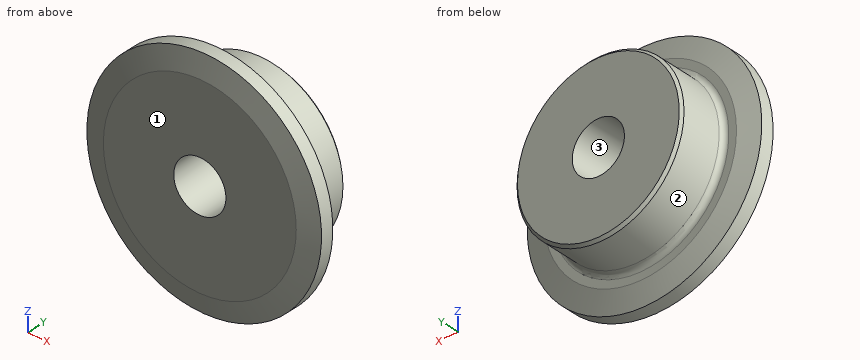
from build123d import *

# Parameters (mm, degrees)
F0_W     = 28.4
F0_H     = 40.5
F0_H_2   = 68.75
F0_W_2   = 59.1
F2_R     = 6.25
F3_SIZE  = 3.125
F4_SIZE2 = 25
F4_SIZE  = 6.2


with BuildPart() as f1:
    # F0 (on Right) → F1 (revolve)
    with BuildSketch(Plane.YZ):
        with Locations((14.2, 120.25)):
            Rectangle(F0_W, F0_H)
        with Locations((14.2, 65.625)):
            Rectangle(F0_W, F0_H_2)
        with Locations((57.95, 65.625)):
            Rectangle(F0_W_2, F0_H_2)
    revolve(axis=Axis((0, 43.75, 0), (0, 1, 0)))

    # F2
    f2_edges = [f1.edges().sort_by_distance(p)[0] for p in [
        (0, 28.4, -100),
    ]]
    fillet(f2_edges, radius=F2_R)

    # F3
    f3_edges = [f1.edges().sort_by_distance(p)[0] for p in [
        (0, 87.5, -100),
    ]]
    chamfer(f3_edges, length=F3_SIZE)

    # F4
    f4_edges = [f1.edges().sort_by_distance(p)[0] for p in [
        (0, 0, -140.5),
        (0, 28.4, -140.5),
    ]]
    f4_side = f1.faces().sort_by_distance((0, 14.2, -140.5))[0]
    chamfer(f4_edges, length=F4_SIZE, length2=F4_SIZE2, reference=f4_side)


solid = f1.part
Check sheet for the modelled part. Datum: model origin and axes. Units: mm. Face numbers are marked on the shaded views. Coordinates: 2 decimals unless noted, no trailing zeros. Write each loop counter-clockwise with the first axis right and the second up, starting at its lowest first coordinate (ties: lowest second). Pieces come first, ordered by that corner, then holes.
Item 1: Cross-section at B-B on z = 0. Record the boundary of the cut face in (x, y) (3 decimals), then the cut area to 3 significant figures.
Numbers:
outline: (-140.5, 6.2) - (-115.5, 0) - (-31.25, 0) - (-31.25, 87.5) - (-96.875, 87.5) - (-100, 84.375) - (-100, 34.65) arc R6.25 cw to (-106.25, 28.4) - (-115.5, 28.4) - (-140.5, 22.2) - close; (31.25, 0) - (115.5, 0) - (140.5, 6.2) - (140.5, 22.2) - (115.5, 28.4) - (106.25, 28.4) arc R6.25 cw to (100, 34.65) - (100, 84.375) - (96.875, 87.5) - (31.25, 87.5) - close
area: 14,000 mm2
Item 2: Mould release check, pull along X, two halves, no side actions. Record for the marked faces 1, 2 and 3: released by +X, released by -X, zero draft, split by the parting line, or undercut.
Numbers:
face 1: zero draft
face 2: split by the parting line
face 3: undercut
Item 3: Depth check by flat-ended pin: pin 1 Ø4 at (y, z) = (78, -92) entering from -X; pin 2 Ø12 at (x, y) = (-22.5, 70.5) entering from +Z; pin 3 Ø3 at (x, z) = (92.5, -83) entering from -Y. Enter the tip coordinate at first touch or a pass-through.
Numbers:
pin 1: stops at x = -43.59
pin 2: stops at z = 98.63
pin 3: stops at y = 1.81
Item 4: Cross-section at C-C on y = 39. Record the boundary of the cut face in (x, z).
Numbers:
outline: circle Ø200 at (0, 0); hole circle Ø62.5 at (0, 0)
Item 5: Scan lines: probe 1 along X at (y, z) = (69, 0); probe 2 along X at (y, z) = (16, 1.5); probe 3 along Y at (x, z) = (58, -121.5). Record each from-to range of solid material in increasing order.
Numbers:
probe 1: x = -100 to -31.25, 31.25 to 100
probe 2: x = -140.49 to -31.21, 31.21 to 140.49
probe 3: y = 4.75 to 23.65
Item 6: Cross-section at A-A on x = 0. Record the boundary of the cut face in (y, z) (3 decimals), then the cut area to 3 significant figures.
Numbers:
outline: (0, -115.5) - (6.2, -140.5) - (22.2, -140.5) - (28.4, -115.5) - (28.4, -106.25) arc R6.25 cw to (34.65, -100) - (84.375, -100) - (87.5, -96.875) - (87.5, -31.25) - (0, -31.25) - close; (0, 31.25) - (87.5, 31.25) - (87.5, 96.875) - (84.375, 100) - (34.65, 100) arc R6.25 cw to (28.4, 106.25) - (28.4, 115.5) - (22.2, 140.5) - (6.2, 140.5) - (0, 115.5) - close
area: 14,000 mm2
